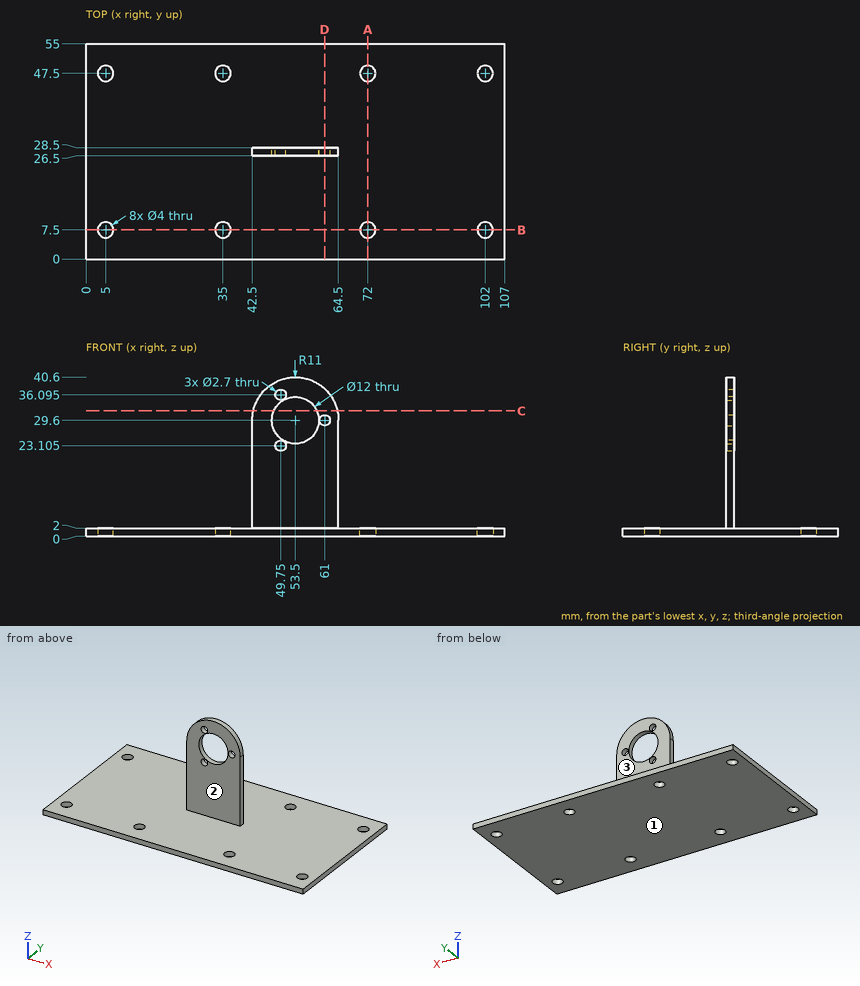
For this review, use the dimensioned drawing (mm, ordinates from the lowest corner) and the shaded views. A direction names the side the tool comes from. Give positions to 0.01 mm unless a question says otherwise; leave off trailing zeros. Order: outer loops, then holes, each group sorted by start corner. A loop starts at its lowest first (then second) coordinate and runs counter-clockwise, first axis right, second up.
1) Take a section at C-C (z = 32). Give the boundary of the cut face in (x, y) (3 decimals).
2) Take a section at A-A (x = 72). Give the boundary of the cut face in (y, z).
3) Take a section at D-D (x = 61). Give the boundary of the cut face in (y, z), then the cut area to 3 significant figures.
4) For the marked faces 1, 2 and 3, list the 3-axis set-ups (+Z, -Z, +X, -X, +Y, -Y) from which the entire face can be reached by the end or side of a thin tool; tool diameter is ignored.
5) Insertion check: pin 1 (0.6 mm diameter, centred on y = 27.5, z = 16, fed in from -X); pin 2 (14 mm diameter, centred on x = 53.5, z = 29.6, fed in from -Y); pin 3 (2.5 mm diameter, centred on x = 5, y = 7.5, fed in from -Z); pin 4 (0.6 mm diameter, centred on y = 27.5, z = 14, fed in from +X). Each pin has a flat end and moves straight along its axis. Give the tip position at first contact, or say it passes through.
6) Take a section at B-B (y = 7.5). Give the boundary of the cut face in (x, z), then the cut area to 3 significant figures.
7) Wall thickness on line 1 (Y direction, x = 102, z = 1); line 2 (X direction, y = 27, z = 29); line 3 (Z direction, x = 67.5, y = 23): over which ranges is each line inside the solid? List them lowest first.
Derived:
1. outline: (42.765, 26.5) - (48.001, 26.5) - (48.001, 28.5) - (42.765, 28.5) - close; (58.999, 26.5) - (64.235, 26.5) - (64.235, 28.5) - (58.999, 28.5) - close
2. outline: (0, 0) - (5.5, 0) - (5.5, 2) - (0, 2) - close; (9.5, 0) - (45.5, 0) - (45.5, 2) - (9.5, 2) - close; (49.5, 0) - (55, 0) - (55, 2) - (49.5, 2) - close
3. outline: (0, 0) - (55, 0) - (55, 2) - (28.5, 2) - (28.5, 28.25) - (26.5, 28.25) - (26.5, 2) - (0, 2) - close; (26.5, 30.95) - (28.5, 30.95) - (28.5, 37.65) - (26.5, 37.65) - close
3. area: 176 mm2
4. face 1: -Z, +X, -X, +Y, -Y
4. face 2: +Z, +X, -X, -Y
4. face 3: +Z, +X, -X, +Y
5. pin 1: stops at x = 42.5
5. pin 2: stops at y = 26.5
5. pin 3: passes through
5. pin 4: stops at x = 64.5
6. outline: (0, 0) - (3, 0) - (3, 2) - (0, 2) - close; (7, 0) - (33, 0) - (33, 2) - (7, 2) - close; (37, 0) - (70, 0) - (70, 2) - (37, 2) - close; (74, 0) - (100, 0) - (100, 2) - (74, 2) - close; (104, 0) - (107, 0) - (107, 2) - (104, 2) - close
6. area: 182 mm2
7. line 1: y = 0 to 5.5, 9.5 to 45.5, 49.5 to 55
7. line 2: x = 42.5 to 47.53, 59.47 to 59.79, 62.21 to 64.5
7. line 3: z = 0 to 2
